```python
from build123d import *

# Parameters (mm, degrees)
F2_R = 1
F3_R = 0.6


# Not quite as in the source:
# - a feature names something its author has since deleted; it is built from what else it names


with BuildPart() as f1:
    # F0 (on Front) → F1 (revolve)
    with BuildSketch(Plane.XZ):
        with BuildLine():
            Line((40, 17.4), (11.5, 17.4))
            Line((11.5, 17.4), (0, 17.4))
            Line((0, 17.4), (0, 15.6))
            Line((0, 15.6), (40, 15.6))
            ThreePointArc((40, 15.6), (46.7596616101, 12.8406114977), (54, 11.9))
            Line((54, 11.9), (54, 17.4))
            Line((54, 17.4), (51, 17.4))
            Line((51, 17.4), (51, 14.4))
            ThreePointArc((51, 14.4), (45.2991228745, 15.1634505398), (40, 17.4))
        make_face()
    revolve(axis=Axis((27, 0, 0), (1, 0, 0)))

    # F2
    f2_edges = [f1.edges().sort_by_distance(p)[0] for p in [
        (54, 0, -17.4),
        (51, 0, -17.4),
    ]]
    fillet(f2_edges, radius=F2_R)

    # F3
    f3_edges = [f1.edges().sort_by_distance(p)[0] for p in [
        (0, 0, -15.6),
    ]]
    fillet(f3_edges, radius=F3_R)


solid = f1.part
```
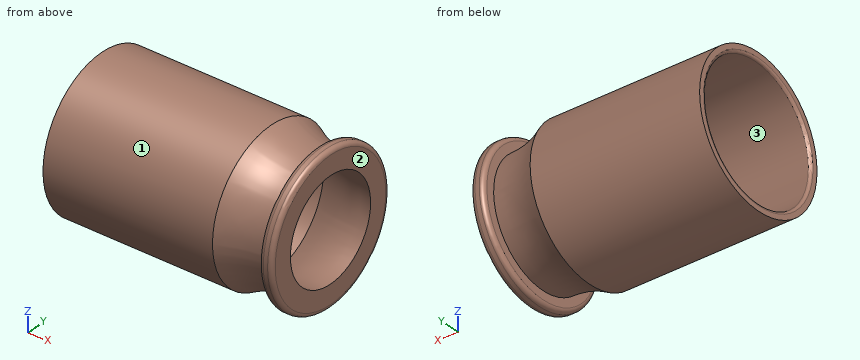
Build history of the part. All positions in model axes, mm. Face numbers are marked on the shaded views. Round coordinates to 2 decimals unless told otherwise and drop trailing zeros. Order: outer loops, then holes, each group sorted by start corner. A loop starts at its lowest first (then second) coordinate and runs counter-clockwise, first axis right, second up. Notation, with made-up numbers: (-16.5, 89.5) -> (29.5, 89.5) arc R23 cw to (29.5, 104.5) -> close; hole circle Ø3 at (-36, 71). An arc over 180 degrees is marked (long way). Answer in a Markdown table with one row per item.
1) Pin check, flat tips, straight feed: P1, Ø5, axis at x = 7, z = 9.5, coming from the +Y side; P2, Ø3, axis at x = 47, y = 6.5, coming from the -Z side; P3, Ø1, axis at x = 8, z = -4, coming from the +Y side. Stop position of each tip, or through.
Values:
| item | result |
|---|---|
| P1 | y = 15.93 |
| P2 | z = -13.99 |
| P3 | y = 17.04 |
2) Wall check: L1, parallel to Y at x = 16, z = 0; L2, parallel to Z at x = 21, y = -5.5. Give the ranges that are in metal, low to high.
Values:
| item | result |
|---|---|
| L1 | -17.4 to -15.6, 15.6 to 17.4 |
| L2 | -16.51 to -14.6, 14.6 to 16.51 |
3) Band-saw the part on D-D on x = 42.5. Give the cut face in (y, z).
Values:
| item | result |
|---|---|
| outline | circle Ø32.27 at (0, 0); hole circle Ø28.68 at (0, 0) |
4) Band-saw the part on A-A on z = 0. Give the cut face in (x, y), and give its area (3 significant figures).
Values:
| item | result |
|---|---|
| outline | (0, -17.4) -> (40, -17.4) arc R21.67 cw to (51, -14.4) -> (51, -16.4) arc R1 ccw to (52, -17.4) -> (53, -17.4) arc R1 ccw to (54, -16.4) -> (54, -11.9) arc R28.34 ccw to (40, -15.6) -> (0.6, -15.6) arc R0.6 ccw to (0, -16.2) -> close; (0, 16.2) arc R0.6 ccw to (0.6, 15.6) -> (40, 15.6) arc R28.34 ccw to (54, 11.9) -> (54, 16.4) arc R1 ccw to (53, 17.4) -> (52, 17.4) arc R1 ccw to (51, 16.4) -> (51, 14.4) arc R21.67 cw to (40, 17.4) -> (0, 17.4) -> close |
| area | 219 mm2 |
5) Band-saw the part on C-C on x = 11. Give the cut face in (y, z), and give its area (3 significant figures).
Values:
| item | result |
|---|---|
| outline | circle Ø34.8 at (0, 0); hole circle Ø31.2 at (0, 0) |
| area | 187 mm2 |
6) Mould opens along Y. For the marked faces 1, 2 and 3 say: released by +Y, released by -Y, zero draft, split by the parting line, or undercut.
Values:
| item | result |
|---|---|
| face 1 | split by the parting line |
| face 2 | zero draft |
| face 3 | undercut |
